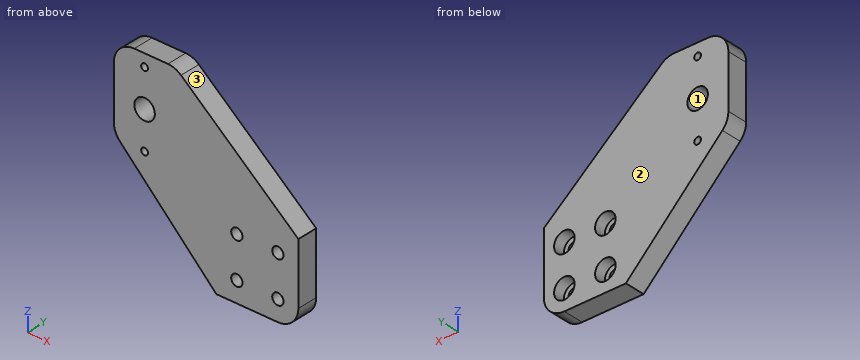
from build123d import *

# Parameters (mm, degrees)
BOSS_EXTRUDE1_DEPTH                                 = 5
CBORE_FOR_M5_HEX_SOCKET_HEAD_CAP_SCREW2_D           = 5.5
CBORE_FOR_M5_HEX_SOCKET_HEAD_CAP_SCREW2_CBORE_D     = 10
CBORE_FOR_M5_HEX_SOCKET_HEAD_CAP_SCREW2_CBORE_DEPTH = 5.5
M4_TAPPED_HOLE1_D                                   = 3.3
SKETCH8_R                                           = 5
CUT_EXTRUDE3_DEPTH                                  = 100.498743711
FILLET1_R                                           = 10


with BuildPart() as part:
    # Sketch1 → Boss-Extrude1 (new, symmetric)
    with BuildSketch(Plane(origin=(0, 0, 0), x_dir=(1, 0, 0), z_dir=(0, 1, 0))):
        Polygon((-20, 20), (20, 20), (20, -20), (-40, -70), (-70, -70), (-70, -30), align=None)
    extrude(amount=BOSS_EXTRUDE1_DEPTH, both=True)

    # CBORE for M5 Hex Socket Head Cap Screw2 (through all)
    with Locations(Plane(origin=(0, 5, 0), x_dir=(1, 0, 0), z_dir=(0, 1, 0))):
        with Locations((-10, 10), (10, 10), (10, -10), (-10, -10)):
            CounterBoreHole(CBORE_FOR_M5_HEX_SOCKET_HEAD_CAP_SCREW2_D / 2, CBORE_FOR_M5_HEX_SOCKET_HEAD_CAP_SCREW2_CBORE_D / 2, CBORE_FOR_M5_HEX_SOCKET_HEAD_CAP_SCREW2_CBORE_DEPTH)

    # M4 Tapped Hole1 (through all)
    with Locations(Plane(origin=(0, 5, 0), x_dir=(1, 0, 0), z_dir=(0, 1, 0))):
        with Locations((-55, -27.5), (-55, -64)):
            Hole(M4_TAPPED_HOLE1_D / 2)

    # Sketch8 → Cut-Extrude3 (cut, through all)
    with BuildSketch(Plane(origin=(0, 5, 0), x_dir=(1, 0, 0), z_dir=(0, 1, 0))):
        with Locations(Location((-55, -45.75, 0), (0, 0, 270))):
            Circle(SKETCH8_R)
    extrude(amount=-CUT_EXTRUDE3_DEPTH, mode=Mode.SUBTRACT)

    # Fillet1
    fillet1_edges = [part.edges().sort_by_distance(p)[0] for p in [
        (20, 0, -20),
        (-40, 0, 70),
        (-70, 0, 70),
        (-70, 0, 30),
    ]]
    fillet(fillet1_edges, radius=FILLET1_R)


solid = part.part
Input: part model. Units: mm. Frame: model coordinates. Face numbers are marked on the shaded views. Give positions to 0.01 mm unless a question says otherwise; leave off trailing zeros. Write each loop counter-clockwise with the first axis right and the second up, starting at its lowest first coordinate (ties: lowest second). Pieces come first, ordered by that corner, then holes.
Q1. Section C-C, the plane y = -3.75. Output: boundary loops of the cut face in (x, z), plus the area to 3 significant figures.
Q2. Section B-B, the plane x = -58. Output: boundary loops of the cut face in (y, z), plus the area to 3 significant figures.
Q3. Section D-D, the plane z = 10. Output: boundary loops of the cut face in (x, y).
Q4. First-contact query: P1, Ø3, axis at x = 12, z = 8.5, coming from the +Y side; P2, Ø1.5, axis at y = 0, z = -4.5, coming from the -X side; P3, Ø4, axis at x = -55, z = 64, coming from the +Y side; P4, Ø6, axis at y = 3, z = 50, coming from the +X side. Flat tips, straight axial feed; report the tip coordinate or a pass-through.
Q5. Pull-direction query (X, two-part tool) for the marked faces 1, 2 and 3; classes: pulls with the +X half, pulls with the -X half, needs draft (parallel to the pull), parting line crosses it, or undercut.
Q6. Section A-A, the plane z = 45.75. Output: boundary loops of the cut face in (x, y), plus the area to 3 significant figures.
Q7. Material intervals for probe 1 along Z at (x, y) = (9.5, -4.5); probe 2 along Z at (x, y) = (-10, -2.7); probe 3 along X at (y, z) = (1.5, -12.5), sorted ascending.
Filled in:
1. outline: (-70, 34.14) arc R10 ccw to (-67.07, 27.07) - (-20, -20) - (10, -20) arc R10 ccw to (20, -10) - (20, 20) - (-37.22, 67.68) arc R10 ccw to (-43.62, 70) - (-60, 70) arc R10 ccw to (-70, 60) - close; hole circle Ø10 at (-55, 45.75); hole circle Ø3.3 at (-55, 27.5); hole circle Ø3.3 at (-55, 64); hole circle Ø5.5 at (-10, -10); hole circle Ø5.5 at (-10, 10); hole circle Ø5.5 at (10, -10); hole circle Ø5.5 at (10, 10)
1. area: 5,110 mm2
2. outline: (-5, 18) - (5, 18) - (5, 41.75) - (-5, 41.75) - close; (-5, 49.75) - (5, 49.75) - (5, 70) - (-5, 70) - close
2. area: 440 mm2
3. outline: (-50, -5) - (-12.75, -5) - (-12.75, -0.5) - (-15, -0.5) - (-15, 5) - (-50, 5) - close; (-7.25, -5) - (7.25, -5) - (7.25, -0.5) - (5, -0.5) - (5, 5) - (-5, 5) - (-5, -0.5) - (-7.25, -0.5) - close; (12.75, -5) - (20, -5) - (20, 5) - (15, 5) - (15, -0.5) - (12.75, -0.5) - close
4. P1: stops at y = -0.5
4. P2: stops at x = -36.25
4. P3: stops at y = 5
4. P4: stops at x = -12.4
5. face 1: undercut
5. face 2: needs draft
5. face 3: pulls with the +X half
6. outline: (-70, -5) - (-60, -5) - (-60, 5) - (-70, 5) - close; (-50, -5) - (-10.9, -5) - (-10.9, 5) - (-50, 5) - close
6. area: 491 mm2
7. probe 1: z = -20 to -12.7, -7.3 to 7.3, 12.7 to 28.75
7. probe 2: z = -20 to -12.75, -7.25 to 7.25, 12.75 to 45
7. probe 3: x = -27.5 to -14.33, -5.67 to 5.67, 14.33 to 19.68
